For this review, take the finished solid that the model builds, in its own axes (mm). Give positions to 0.01 mm unless a question says otherwise; leave off trailing zeros. Write each loop counter-clockwise with the first axis right and the second up, starting at its lowest first coordinate (ties: lowest second). Pieces come first, ordered by that corner, then holes.
Q1. We need section A-A (y = -4.5). Write out the cut boundary in (x, z), then the cut area to 3 significant figures.
Q2. We need section B-B (z = 360). Write out the cut boundary in (x, y).
Q3. Insertion check: P1, Ø4, axis at x = 8.5, y = 5, coming from the +Z side; P2, Ø10, axis at x = 7.5, y = -8, coming from the +Z side. Each pin has a flat end and moves straight along its axis. Give the tip position at first contact, or say it passes through.
Q4. For line 1 (Y direction, x = -1, z = 1146.5); line 2 (Y direction, x = 10, z = 534.5), list the stretches that pass through material, from the lowest coordinate up.
Q5. We need section C-C (x = 2.5). Write out the cut boundary in (y, z).
Autodesk Inventor part; units mm, degrees
ref_plane "Start Plane" through (0, 0, 19.7356) normal (0, 0, 1) x (1, 0, 0)
ref_plane "End Plane" through (0, 0, 1295.0132) normal (0, 0, 1) x (1, 0, 0)
ref_plane "Work Plane4" through (-472.3083, -9, 221.6126) normal (-0.3986, 0, -0.9171) x (-0.9171, 0, 0.3986)
ref_plane "Start Plane" through (0, 0, 19.7356) normal (0, 0, 1) x (1, 0, 0)
ref_plane "End Plane" through (0, 0, 1295.0132) normal (0, 0, 1) x (1, 0, 0)
sketch "Sketch" plane through (0, 0, 0) normal (0, 0, 1) x (1, 0, 0)
  line L0 (-15, -9) -> (-15, 9)
  line L1 (-9, 15) -> (9, 15)
  line L2 (15, 9) -> (15, -9)
  line L3 (9, -15) -> (-9, -15)
  arc A0 (-15, -9) -> (-9, -15) centre (-9, -9) ccw
  arc A1 (-9, 15) -> (-15, 9) centre (-9, 9) ccw
  arc A2 (15, 9) -> (9, 15) centre (9, 9) ccw
  arc A3 (9, -15) -> (15, -9) centre (9, -9) ccw
  arc A4 (-9, 12) -> (-12, 9) centre (-9, 9) ccw
  line L4 (-9, 12) -> (9, 12)
  arc A5 (12, 9) -> (9, 12) centre (9, 9) ccw
  line L5 (12, 9) -> (12, -9)
  arc A6 (9, -12) -> (12, -9) centre (9, -9) ccw
  line L6 (9, -12) -> (-9, -12)
  arc A7 (-12, -9) -> (-9, -12) centre (-9, -9) ccw
  line L7 (-12, -9) -> (-12, 9)
  line L8 (0, 22.7397) -> (0, -22.7397) construction
  line L9 (-22.7397, 0) -> (22.7397, 0) construction
  dimension "d7" = 6
  dimension "d10" = 30
  dimension "d11" = 30
  dimension "d12" = 3
  dimension "d15" = 15
  dimension "d16" = 15
extrude "Body" add sketch "Sketch" along normal up to surface (1275.2776 mm away) from surface at 19.7356
sketch "Sketch3" plane through (0, 0, 0) normal (0, 0, 1) x (1, 0, 0)
  line L0 (0, 0) -> (10, 0)
ref_plane "Work Plane3" through (0, 0, 0) normal (0, -1, 0) x (1, 0, 0)
ref_plane "Work Plane4" through (-472.3083, -9, 221.6126) normal (-0.3986, 0, -0.9171) x (-0.9171, 0, 0.3986)
split "Split1" plane through (-472.3083, -9, 221.6126) removes the side toward (-0.3986, 0, -0.9171)
ref_plane "Work Plane5" through (-13.7571, -9, 5.9786) normal (0.9171, 0, -0.3986) x (-0.3986, 0, -0.9171)
split "Split2" plane through (-13.7571, -9, 5.9786) removes the side toward (0.9171, 0, -0.3986)
ref_plane "Work Plane6" through (13.7571, -9, 1302.4412) normal (-0.9171, 0, 0.3986) x (0.3986, 0, 0.9171)
split "Split3" plane through (13.7571, -9, 1302.4412) removes the side toward (-0.9171, 0, 0.3986)
ref_plane "Work Plane7" through (1.6776, 9, 1293.5139) normal (-0.1118, 0, 0.9937) x (0.9937, 0, 0.1118)
split "Split4" plane through (1.6776, 9, 1293.5139) removes the side toward (-0.1118, 0, 0.9937)
sketch "Sketch4" plane through (0, 0, 0) normal (0, -1, 0) x (1, 0, 0)
  line L0 (-2, 19.7356) -> (12, 19.7356)
  line L1 (-2, 1295.0132) -> (12, 1295.0132)
  dimension "d18" = 1275.2776
equation "\"d7\" = G_IR"
equation "\"d10\" = G_H"
equation "\"d11\" = G_W"
equation "\"d12\" = G_T"
equation "\"d15\" = 0.5 * d10"
equation "\"d16\" = 0.5 * d11"
equation "\"d3\" = G_L"
equation "\"G_W\" = 30"
equation "\"G_H\" = 30"
equation "\"G_T\" = 3"
equation "\"G_IR\" = 6"
equation "\"G_L\" = d18"
equation "\"G_OFFSET_START\" = -19.73564"
equation "\"G_OFFSET_END\" = -13.40653"
equation "\"d13\" = -G_OFFSET_START"
equation "\"d14\" = G_OFFSET_END + B_L"
equation "\"B_L\" = 1308.41975"
properties part number "DIN EN 10219-2 - 30 x 30 x 3  - 1275.28" material "Steel, Mild"
Computed:
1. outline: (-15, 22.85) - (-12, 21.55) - (-12, 1243.18) - (-15, 1236.28) - close; (12, 65.24) - (15, 72.14) - (15, 1295.01) - (12, 1294.68) - close
1. area: 7,330 mm2
2. outline: (-15, -9) arc R6 ccw to (-9, -15) - (9, -15) arc R6 ccw to (15, -9) - (15, 9) arc R6 ccw to (9, 15) - (-9, 15) arc R6 ccw to (-15, 9) - close; hole (-12, -9) arc R3 ccw to (-9, -12) - (9, -12) arc R3 ccw to (12, -9) - (12, 9) arc R3 ccw to (9, 12) - (-9, 12) arc R3 ccw to (-12, 9) - close
3. P1: passes through
3. P2: stops at z = 1294.73
4. line 1: y = -15 to -12, 12 to 15
4. line 2: y = -14.92 to -11.83, 11.83 to 14.92
5. outline: (-15, 43.38) - (-12, 43.38) - (-12, 1276.54) - (-15, 1276.54) - close; (12, 43.38) - (15, 43.38) - (15, 1276.54) - (12, 1276.54) - close
